Autodesk Inventor part; units mm, degrees
ref_plane "YZ Plane" through (0, 0, 0) normal (1, 0, 0) x (0, 1, 0)
ref_plane "XZ Plane" through (0, 0, 0) normal (0, 1, 0) x (-1, 0, 0)
ref_plane "XY Plane" through (0, 0, 0) normal (0, 0, 1) x (1, 0, 0)
sketch "スケッチ1" plane through (0, 0, 0) normal (0, 0, 1) x (1, 0, 0)
  line L0 (0, 0) -> (70, 0)
  line L1 (70, 0) -> (70, 70)
  line L2 (70, 70) -> (0, 70)
  line L3 (0, 70) -> (0, 0)
  dimension "d0" = 70
  dimension "d1" = 70
extrude "押し出し1" add sketch "スケッチ1" along normal blind 10
sketch "スケッチ2" plane through (0, 0, 10) normal (0, 0, 1) x (1, 0, 0)
  line L0 (70, 70) -> (0, 70)
  line L1 (70, 0) -> (70, 70)
  line L2 (0, 0) -> (70, 0)
  line L3 (35, 70) -> (35, 0)
  point P0 (40, 65)
  point P1 (65, 40)
  point P2 (65, 30)
  point P3 (40, 5)
  point P4 (30, 65)
  point P5 (5, 40)
  point P6 (5, 30)
  point P7 (30, 5)
  dimension "d4" = 5
  dimension "d5" = 5
  dimension "d6" = 5
  dimension "d7" = 5
  dimension "d8" = 30
  dimension "d9" = 30
  dimension "d10" = 30
  dimension "d11" = 30
hole "穴1" at (40, 65, 10) at (65, 40, 10) at (65, 30, 10) at (40, 5, 10) at (30, 65, 10) at (5, 40, 10) at (5, 30, 10) at (30, 5, 10) direction (0, 0, -1) diameter 3.5 end through all counterbore diameter 6 counterbore depth 4
sketch "スケッチ10" plane through (0, 0, 10) normal (0, 0, 1) x (1, 0, 0)
  line L0 (0, 70) -> (0, 0)
  line L1 (70, 70) -> (0, 70)
  line L2 (0, 0) -> (70, 70)
  line L3 (70, 0) -> (70, 70)
  line L4 (70, 0) -> (0, 70)
  point P0 (10.2513, 59.7487)
  point P1 (59.7487, 10.2513)
  point P2 (10.2513, 10.2513)
  point P3 (59.7487, 59.7487)
  dimension "d41" = 70
  dimension "d42" = 70
hole "穴3" at (10.2513, 59.7487, 10) at (59.7487, 10.2513, 10) at (10.2513, 10.2513, 10) at (59.7487, 59.7487, 10) direction (0, 0, -1) diameter 3.5 end through all
sketch "スケッチ13" plane through (0, 0, 10) normal (0, 0, 1) x (1, 0, 0)
  line L0 (0, 70) -> (0, 0)
  line L1 (0, 0) -> (70, 0)
  line L2 (0, 70) -> (70, 0)
  line L3 (70, 70) -> (0, 70)
  line L4 (70, 70) -> (0, 0)
  point P0 (23.6863, 37.8284)
  point P1 (37.8284, 23.6863)
  point P2 (32.1716, 46.3137)
  point P3 (46.3137, 32.1716)
  dimension "d85" = 12
  dimension "d86" = 20
  dimension "d89" = 20
  dimension "d92" = 12
hole "穴6" at (23.6863, 37.8284, 10) at (37.8284, 23.6863, 10) at (32.1716, 46.3137, 10) at (46.3137, 32.1716, 10) direction (0, 0, -1) diameter 1.567 end through all
properties part number "土台"
Part model, mm, in its own coordinate system. A direction names the side the tool comes from. Give positions to 0.01 mm unless a question says otherwise; leave off trailing zeros. Loops run counter-clockwise (first coordinate to the right, second up) from the corner with the lowest first, then second, coordinate; pieces in that order, holes last. Notation, with made-up numbers: M 84.25,-33 L 133.25,-33 A21 ccw 133.25,-4 Z; hole C 34,3 d5. An arc over 180 degrees is marked long. Return JSON: item names as keys, results as strings.
1) Pull direction Y, two halves, no side cores. Call faces 3 (the face through (35, 70, 5)), 4 (the face through (0, 35, 5)), 5 (the face through (66.55, 39.19, 2.96)): released by +Y, released by -Y, zero draft, split by the parting line, or undercut.
Calculated:
{"face 3": "released by +Y", "face 4": "zero draft", "face 5": "undercut"}
2) Flat gauge pins, fed straight in: pin 1 Ø4.5 at (x, y) = (40, 5) entering from +Z; pin 2 Ø3 at (x, y) = (65, 30) entering from -Z. Where does each tip first touch, or does it go through?
Calculated:
{"pin 1": "stops at z = 6", "pin 2": "passes through"}
3) Saw through at A-A, the plane y = 40. List the corners of the cut face in (x, z), then the cut area to 3 significant figures.
Calculated:
{"outline": "M 0,0 L 3.25,0 L 3.25,6 L 2,6 L 2,10 L 0,10 Z; M 6.75,0 L 63.25,0 L 63.25,6 L 62,6 L 62,10 L 8,10 L 8,6 L 6.75,6 Z; M 66.75,0 L 70,0 L 70,10 L 68,10 L 68,6 L 66.75,6 Z", "area": "610 mm2"}
4) Saw through at C-C, the plane z = 8. Count the separate pieces of the cut face and the enclosed holes in it, then the cut area to 3 significant figures.
Calculated:
{"separate pieces": "1", "enclosed holes": "16", "area": "4,630 mm2"}
5) Drill centre lines: line 1 (X direction, y = 40, z = 3.5); line 2 (Y direction, x = 65, z = 7.1); line 3 (Y direction, x = 10.5, z = 1.75). Where is each one in solid material? Low to high.
Calculated:
{"line 1": "x = 0 to 3.25, 6.75 to 63.25, 66.75 to 70", "line 2": "y = 0 to 27, 33 to 37, 43 to 70", "line 3": "y = 0 to 8.52, 11.98 to 58.02, 61.48 to 70"}
6) 3-axis set-ups, long thin cutter, end or side, ignore diameter. For faces 1 (the face through (66.8, 32.4, 8)), 2 (the face through (31.55, 4.19, 2.96)): which of +Z, -Z, +X, -X, +Y, -Y reach the whole face in a straight line?
Calculated:
{"face 1": "+Z", "face 2": "+Z, -Z"}
